```python
from build123d import *

# Parameters (mm, degrees)
SZKIC1_W                    = 200
SZKIC1_H                    = 5
SZKIC1_W_2                  = 46
SZKIC1_H_2                  = 37
SZKIC1_W_3                  = 24
SZKIC1_W_4                  = 125
DODANIE_WYCI_GNI_CIE1_DEPTH = 5


with BuildPart() as part:
    # Szkic1 → Dodanie-wyciągnięcie1 (new body)
    with BuildSketch(Plane(origin=(0, 0, 0), x_dir=(1, 0, 0), z_dir=(0, 1, 0))):
        with Locations((-8.765553919, -32.5)):
            Rectangle(SZKIC1_W, SZKIC1_H)
        with Locations((44.234446081, 91.5)):
            Rectangle(SZKIC1_W_2, SZKIC1_H_2)
        with Locations((79.234446081, 91.5)):
            Rectangle(SZKIC1_W_3, SZKIC1_H_2)
        with Locations((-46.265553919, 75.5)):
            Rectangle(SZKIC1_W_4, SZKIC1_H)
        Polygon((16.234446081, 73), (21.234446081, 73), (21.234446081, 110), (21.234446081, 115), (16.234446081, 115), (16.234446081, 78), align=None)
        Polygon((67.234446081, 110), (91.234446081, 110), (91.234446081, 115), (21.234446081, 115), (21.234446081, 110), align=None)
        with BuildLine():
            Line((91.234446081, -30), (91.234446081, 21.5))
            Line((91.234446081, 21.5), (70.234446081, 21.5))
            ThreePointArc((70.234446081, 21.5), (65.113125737, 19.378679656), (67.234446081, 24.5))
            Line((67.234446081, 24.5), (67.234446081, 73))
            Line((67.234446081, 73), (21.234446081, 73))
            Line((21.234446081, 73), (16.234446081, 73))
            Line((16.234446081, 73), (-108.765553919, 73))
            Line((-108.765553919, 73), (-108.765553919, -30))
            Line((-108.765553919, -30), (91.234446081, -30))
        make_face()
        with BuildLine():
            Line((70.234446081, 21.5), (91.234446081, 21.5))
            Line((91.234446081, 21.5), (91.234446081, 73))
            Line((91.234446081, 73), (67.234446081, 73))
            Line((67.234446081, 73), (67.234446081, 24.5))
            ThreePointArc((67.234446081, 24.5), (69.355766424, 23.621320344), (70.234446081, 21.5))
        make_face()
    extrude(amount=-DODANIE_WYCI_GNI_CIE1_DEPTH)


solid = part.part
```
Input: part model. Units: mm. Frame: model coordinates. A direction names the side the tool comes from. Give positions to 0.01 mm unless a question says otherwise; leave off trailing zeros. Order: outer loops, then holes, each group sorted by start corner. A loop starts at its lowest first (then second) coordinate and runs counter-clockwise, first axis right, second up.
1. Set-up query: faces 1 (the face through (-108.766, -2, -22)), 2 (the face through (-47, -2, -78)). Return all of +Z, -Z, +X, -X, +Y, -Y with unobstructed straight access to the full face (end or side cutting, diameter ignored); none if empty.
Computed:
face 1: +Z, -Z, -X, +Y, -Y
face 2: -Z, -X, +Y, -Y
2. Line query: probe 1 along X at (y, z) = (-2.35, -21.5); probe 2 along Z at (x, y) = (-47.5, -4.6); probe 3 along Z at (x, y) = (65, -3.4). Output: solid intervals per line, ascending.
Computed:
probe 1: x = -108.77 to 64.23, 70.23 to 91.23
probe 2: z = -78 to 35
probe 3: z = -115 to -23.5, -19.5 to 35
3. Pin query (flat end, axial travel): pin 1 Ø12 at (x, z) = (-74.5, -67.5) entering from +Y; pin 2 Ø2 at (x, y) = (-24.5, -2.5) entering from -Z. Return the tip coordinate at first contact, or that it passes through.
Computed:
pin 1: stops at y = 0
pin 2: stops at z = -78
4. Cut plane B-B (x = -17). Return loops of the section in (y, z).
Computed:
outline: (-5, -78) - (0, -78) - (0, 35) - (-5, 35) - close
5. Cut plane A-A (y = -2.4). Return loops of the section in (x, z).
Computed:
outline: (-108.77, -78) - (16.23, -78) - (16.23, -115) - (91.23, -115) - (91.23, 35) - (-108.77, 35) - close; hole circle Ø6 at (67.23, -21.5)
